Input: dimensioned drawing with shaded views. Units: mm. Origin: part minimum x, y, z. Coordinates: 2 decimals unless noted, no trailing zeros. Order: outer loops, then holes, each group sorted by start corner. A loop starts at its lowest first (then second) coordinate and runs counter-clockwise, first axis right, second up. Notation, with made-up numbers: M 72,12 L 117,12 A25 cw 117,26 Z; hole C 67,-14.5 d1. An arc over 180 degrees is marked long. Write item = value, one per line.
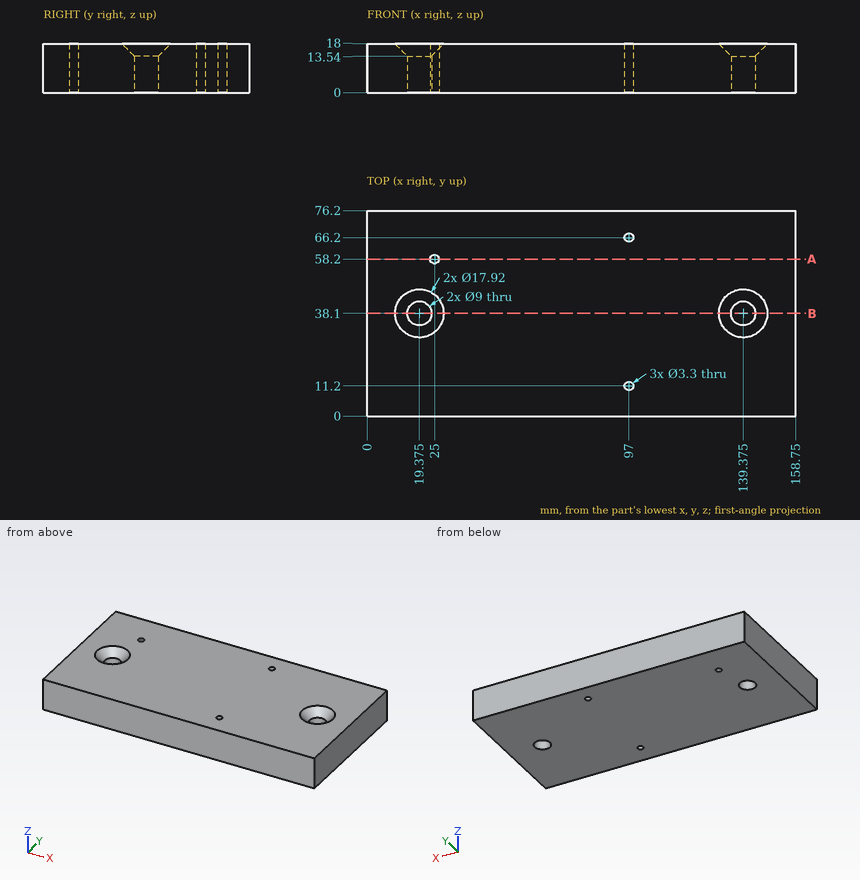
1) Section A-A, the plane y = 58.2. Return loops of the section in (x, z).
Numbers:
outline = M 0,0 L 23.35,0 L 23.35,18 L 0,18 Z; M 26.65,0 L 158.75,0 L 158.75,18 L 26.65,18 Z
2) Section B-B, the plane y = 38.1. Return loops of the section in (x, z) (3 decimals).
Numbers:
outline = M 0,0 L 14.875,0 L 14.875,13.54 L 10.415,18 L 0,18 Z; M 23.875,0 L 134.875,0 L 134.875,13.54 L 130.415,18 L 28.335,18 L 23.875,13.54 Z; M 143.875,0 L 158.75,0 L 158.75,18 L 148.335,18 L 143.875,13.54 Z
3) Line query: L1, parallel to X at y = 38, z = 1.25; L2, parallel to Y at x = 97, z = 13; L3, parallel to Y at x = 25, z = 5.75. Output: solid intervals per line, ascending.
Numbers:
L1 = 0 to 14.88, 23.87 to 134.88, 143.87 to 158.75
L2 = 0 to 9.55, 12.85 to 64.55, 67.85 to 76.2
L3 = 0 to 56.55, 59.85 to 76.2
